Here's how the part is built. I have some questions about the finished solid (model axes, mm). A direction names the side the tool comes from. Round coordinates to 2 decimals unless told otherwise and drop trailing zeros. Loops run counter-clockwise (first coordinate to the right, second up) from the corner with the lowest first, then second, coordinate; pieces in that order, holes last. Notation, with made-up numbers: M 87,18.5 L 97,18.5 A35 cw 97,54.5 Z; hole C -32,70.25 d7. An arc over 180 degrees is marked long. Answer as a JSON object with one key per item and string values.
Autodesk Inventor part; units mm, degrees
ref_plane "YZ Plane" through (0, 0, 0) normal (1, 0, 0) x (0, 1, 0)
ref_plane "XZ Plane" through (0, 0, 0) normal (0, 1, 0) x (-1, 0, 0)
ref_plane "XY Plane" through (0, 0, 0) normal (0, 0, 1) x (1, 0, 0)
sketch "Sketch1" plane through (0, 0, 0) normal (0, 0, 1) x (1, 0, 0)
  circle A0 centre (0, 0) radius 3.6
  line L0 (0, 0) -> (15.95, 0) construction
  circle A1 centre (15.95, 0) radius 2.4
  line L1 (0.2708, 3.5898) -> (16.1306, 2.3932)
  line L2 (0.2708, -3.5898) -> (16.1306, -2.3932)
  line L3 (5.6, 3.1877) -> (5.6, -3.1877)
  line L4 (0, 0) -> (-3.6, 0) construction
  circle A2 centre (0, 0) radius 1.55
  circle A3 centre (15.95, 0) radius 0.85
  circle A4 centre (0, 0) radius 2.975
  dimension "d0" = 7.2
  dimension "d1" = 4.8
  dimension "d2" = 15.95
  dimension "d5" = 9.2
  dimension "d6" = 3.1
  dimension "d7" = 1.7
  dimension "d10" = 5.95
extrude "Extrusion1" add sketch "Sketch1" along normal blind 2 contours A0 | A0 L1 L3 L2 | L1 A1 L2 L3 | A1 | A4
extrude "Extrusion2" add sketch "Sketch1" against normal blind 1.15 contours A0 | A0 L1 L3 L2 | A4
extrude "Extrusion3" add sketch "Sketch1" along normal blind 4 contours A0
chamfer "Chamfer1" distance 1 angle 45 1 edges at (5.6, 0, -1.15)
properties part number "HalfServoArm"
Item 1: I want a section at C-C on z = 1.7. List the corners of the cut face in (x, y) for me.
Solution:
{"outline": "M 0.27,-3.59 L 16.13,-2.39 A2.4 ccw 16.13,2.39 L 0.27,3.59 A3.6 ccw long Z; hole C 0,0 d3.1; hole C 15.95,0 d1.7"}
Item 2: I want a section at D-D on y = -1.75. List the corners of the cut face in (x, z) for me, plus the area to 3 significant figures.
Solution:
{"outline": "M -3.15,-1.15 L 4.6,-1.15 L 5.6,-0.15 L 5.6,0 L 17.59,0 L 17.59,2 L 3.15,2 L 3.15,4 L 2.41,4 L 2.41,2 L -2.41,2 L -2.41,4 L -3.15,4 Z", "area": "54.0 mm2"}
Item 3: For P1, Ø1.5, axis at x = 16, y = 0, coming from the +Z side; P2, Ø2, axis at x = 6.5, z = 2.5, coming from the -Y side; P3, Ø4, axis at x = 0, y = 0, coming from the +Z side; P4, Ø1.5, axis at x = 13, z = -0.5, coming from the +Y side, each with a flat end and sliding along its axis, tell me the tip position at first contact or that it passes through.
Solution:
{"P1": "passes through", "P2": "stops at y = -3.19", "P3": "stops at z = 2", "P4": "stops at y = 2.67"}
Item 4: For faces 1 (the face through (1.3, -1.3, 2)), 2 (the face through (10, 0, 0)), 3 (the face through (0.715, 1.375, 0.403)), which set-ups out of +Z, -Z, +X, -X, +Y, -Y let a thin tool reach every point of the face, with its end or its side?
Solution:
{"face 1": "+Z", "face 2": "-Z, +X, +Y, -Y", "face 3": "+Z, -Z"}
Item 5: I want a section at B-B on x = 0. List the corners of the cut face in (y, z) for me (3 decimals), plus the area to 3 significant figures.
Solution:
{"outline": "M -3.6,-1.15 L -1.55,-1.15 L -1.55,2 L -2.975,2 L -2.975,4 L -3.6,4 Z; M 1.55,-1.15 L 3.6,-1.15 L 3.6,4 L 2.975,4 L 2.975,2 L 1.55,2 Z", "area": "15.4 mm2"}
Item 6: I want a section at A-A on y = 0. List the corners of the cut face in (x, z) for me (3 decimals), plus the area to 3 significant figures.
Solution:
{"outline": "M -3.6,-1.15 L -1.55,-1.15 L -1.55,2 L -2.975,2 L -2.975,4 L -3.6,4 Z; M 1.55,-1.15 L 4.6,-1.15 L 5.6,-0.15 L 5.6,0 L 15.1,0 L 15.1,2 L 3.6,2 L 3.6,4 L 2.975,4 L 2.975,2 L 1.55,2 Z; M 16.8,0 L 18.35,0 L 18.35,2 L 16.8,2 Z", "area": "43.3 mm2"}
Item 7: If I drill on L1, parallel to Y at x = 0, z = 1.05; L2, parallel to Y at x = 0, z = 2.55 (3 decimals); L3, parallel to Z at x = 10.5, y = -2.5, over which ranges is the centre line in solid material (lowest first)? Write a range as from..to.
Solution:
{"L1": "y = -3.6..-1.55, 1.55..3.6", "L2": "y = -3.6..-2.975, 2.975..3.6", "L3": "z = 0..2"}
